```python
from build123d import *

# Parameters (mm, degrees)
SKETCH1_W           = 40
SKETCH1_H           = 34
BOSS_EXTRUDE1_DEPTH = 20
SKETCH2_W           = 13.75
SKETCH2_H           = 3
CUT_EXTRUDE1_DEPTH  = 21
SKETCH3_R           = 9.25
SKETCH3_R_2         = 3.05
BOSS_EXTRUDE2_DEPTH = 3.75
SKETCH4_W           = 7
SKETCH4_H           = 3.7
BOSS_EXTRUDE3_DEPTH = 13.2
SKETCH8_R           = 3.05
BOSS_EXTRUDE5_DEPTH = 8.5


with BuildPart() as part:
    # Sketch1 → Boss-Extrude1 (new body)
    with BuildSketch(Plane(origin=(0, 0, 0), x_dir=(1, 0, 0), z_dir=(0, 1, 0))):
        with Locations((-0.96024493, -2.107462687)):
            Rectangle(SKETCH1_W, SKETCH1_H)
    extrude(amount=BOSS_EXTRUDE1_DEPTH)

    # Sketch2 → Cut-Extrude1 (cut, through all)
    with BuildSketch(Plane(origin=(0, 20, 0), x_dir=(1, 0, 0), z_dir=(0, 1, 0))):
        with Locations((-14.08524493, 13.392537313)):
            Rectangle(SKETCH2_W, SKETCH2_H)
    extrude(amount=-CUT_EXTRUDE1_DEPTH, mode=Mode.SUBTRACT)

    # Sketch3 → Boss-Extrude2 (add)
    with BuildSketch(Plane(origin=(0, 0, -14.892537313), x_dir=(-1, 0, 0), z_dir=(0, 0, -1))):
        with Locations((-9.03975507, 10)):
            Circle(SKETCH3_R)
        with Locations((-9.03975507, 10)):
            Circle(SKETCH3_R_2, mode=Mode.SUBTRACT)
    extrude(amount=BOSS_EXTRUDE2_DEPTH)

    # Sketch4 → Boss-Extrude3 (add)
    with BuildSketch(Plane(origin=(0, 20, 0), x_dir=(1, 0, 0), z_dir=(0, 1, 0))):
        with Locations((-24.46024493, 9.342537313)):
            Rectangle(SKETCH4_W, SKETCH4_H)
        with Locations((22.53975507, 9.342537313)):
            Rectangle(SKETCH4_W, SKETCH4_H)
    extrude(amount=-BOSS_EXTRUDE3_DEPTH)

    # Sketch8 → Boss-Extrude5 (add)
    with BuildSketch(Plane(origin=(0, 0, -14.892537313), x_dir=(-1, 0, 0), z_dir=(0, 0, -1))):
        with Locations((-9.03975507, 10)):
            Circle(SKETCH8_R)
    extrude(amount=BOSS_EXTRUDE5_DEPTH)


solid = part.part
```
The model under review builds one solid part; all positions refer to its coordinate system, in mm. A direction names the side the tool comes from. Coordinates: 2 decimals unless noted, no trailing zeros. Write each loop counter-clockwise with the first axis right and the second up, starting at its lowest first coordinate (ties: lowest second). Pieces come first, ordered by that corner, then holes. Notation, with made-up numbers: (88.25, 59.25) - (106.25, 59.25) arc R8 cw to (106.25, 63.25) - close; hole circle Ø11 at (12.5, 3.25). An arc over 180 degrees is marked (long way). Write item = value, one per line.
(1) Consider section D-D, the plane y = 4.75. Give the boundary of the cut face in (x, z), then the cut area to 3 significant figures.
Result sheet:
outline = (-20.96, -11.89) - (-7.21, -11.89) - (-7.21, -14.89) - (1.42, -14.89) - (1.42, -18.64) - (16.66, -18.64) - (16.66, -14.89) - (19.04, -14.89) - (19.04, 19.11) - (-20.96, 19.11) - close
area = 1,380 mm^2
(2) For P1, Ø7, axis at x = -12.5, y = 14.5, coming from the -Z side; P2, Ø5.5, axis at x = 24, y = 12.5, coming from the -Z side; P3, Ø1.8, axis at x = 24, z = -9, coming from the -Y side, all flat-tipped, find the tip position at first contact; note any pin that passes through.
Result sheet:
P1 = -11.89
P2 = -11.19
P3 = 6.8
(3) Consider section C-C, the plane x = 5. Give the boundary of the cut face in (y, z), then the cut area to 3 significant figures.
Result sheet:
outline = (0, -14.89) - (1.68, -14.89) - (1.68, -18.64) - (18.32, -18.64) - (18.32, -14.89) - (20, -14.89) - (20, 19.11) - (0, 19.11) - close
area = 742 mm^2
(4) Machinability: for faces 1 (the face through (-25, 6.8, -9)), 2 (the face through (-25, 13, -11.193)), 3 (the face through (11.04, 0.97, -16.74)), which of the approach directions +Z, -Z, +X, -X, +Y, -Y give a long, thin tool a straight path to every point of the face, cutting with its end or side? Answer none if there is none.
Result sheet:
face_1 = +Z, -Z, -X, -Y
face_2 = -Z, -X, +Y, -Y
face_3 = -Z
(5) For line 1 (Z direction, x = -19, y = 13); line 2 (X direction, y = 16.75, z = -6); line 3 (Z direction, x = 15.5, y = 9.25), list the stretches that pass through material, from the lowest coordinate up. Write a range as [from, to].
Result sheet:
line_1 = [-11.89, 19.11]
line_2 = [-20.96, 19.04]
line_3 = [-18.64, 19.11]
(6) Consider section B-B, the plane y = 10. Give the boundary of the cut face in (x, z), then the cut area to 3 significant figures.
Result sheet:
outline = (-27.96, -11.19) - (-20.96, -11.19) - (-20.96, -11.89) - (-7.21, -11.89) - (-7.21, -14.89) - (-0.21, -14.89) - (-0.21, -18.64) - (5.99, -18.64) - (5.99, -23.39) - (12.09, -23.39) - (12.09, -18.64) - (18.29, -18.64) - (18.29, -14.89) - (19.04, -14.89) - (19.04, -11.19) - (26.04, -11.19) - (26.04, -7.49) - (19.04, -7.49) - (19.04, 19.11) - (-20.96, 19.11) - (-20.96, -7.49) - (-27.96, -7.49) - close
area = 1,470 mm^2
(7) Consider section A-A, the plane z = -9. Give the boundary of the cut face in (x, y).
Result sheet:
outline = (-27.96, 6.8) - (-20.96, 6.8) - (-20.96, 0) - (19.04, 0) - (19.04, 6.8) - (26.04, 6.8) - (26.04, 20) - (-27.96, 20) - close
